For this review, take the finished solid that the model builds, in its own axes (mm). Coordinates: 2 decimals unless noted, no trailing zeros. Loops run counter-clockwise (first coordinate to the right, second up) from the corner with the lowest first, then second, coordinate; pieces in that order, holes last.
1. Take a section at C-C, the plane x = 12. State the section outline as (y, z) points.
2. Take a section at A-A, the plane x = -12.7. State the section outline as (y, z) points.
3. Clearance check with a flat-ended pin moving along its axis: P1, Ø5, axis at x = -12.7, y = -23.3, coming from the +Z side. State where the tip first meets the part, or that it passes through.
4. Take a section at B-B, the plane z = 1.9. State the section outline as (x, y) points, then the cut area to 3 significant figures.
5. To check wall thickness, follow probe 1 along Y at (x, z) = (-12.7, 1.7); probe 2 along X at (y, z) = (24, 2.3). State the ranges of each line that lie inside material, in increasing order.
Autodesk Inventor part; units mm, degrees
ref_plane "YZ Plane" through (0, 0, 0) normal (1, 0, 0) x (0, 1, 0)
ref_plane "XZ Plane" through (0, 0, 0) normal (0, 1, 0) x (-1, 0, 0)
ref_plane "XY Plane" through (0, 0, 0) normal (0, 0, 1) x (1, 0, 0)
sketch "Sketch1" plane through (0, 0, 0) normal (0, 0, 1) x (1, 0, 0)
  line L0 (-19.05, -36.0045) -> (19.05, -36.0045)
  line L1 (19.05, -36.0045) -> (19.05, 36.0045)
  line L2 (19.05, 36.0045) -> (-19.05, 36.0045)
  line L3 (-19.05, 36.0045) -> (-19.05, -36.0045)
  line L4 (-19.05, -36.0045) -> (19.05, 36.0045) construction
  line L5 (19.05, -36.0045) -> (-19.05, 36.0045) construction
  point P0 (0, 0)
  dimension "d0" = 38.1
  dimension "d1" = 72.009
extrude "Extrusion1" add sketch "Sketch1" along normal blind 2.54
sketch "Sketch2" plane through (0, 0, 2.54) normal (0, 0, 1) x (1, 0, 0)
  circle A0 centre (-12.7, 23.3045) radius 1.85
  circle A1 centre (12.7, 23.3045) radius 1.85
  circle A2 centre (-12.7, -23.3045) radius 1.85
  circle A3 centre (12.7, -23.3045) radius 1.85
  point P0 (0, 0)
extrude "Extrusion2" cut sketch "Sketch2" against normal blind 2.54
properties part number "GearPlate"
Results list:
1. outline: (-36, 0) - (-25.02, 0) - (-25.02, 2.54) - (-36, 2.54) - close; (-21.59, 0) - (21.59, 0) - (21.59, 2.54) - (-21.59, 2.54) - close; (25.02, 0) - (36, 0) - (36, 2.54) - (25.02, 2.54) - close
2. outline: (-36, 0) - (-25.15, 0) - (-25.15, 2.54) - (-36, 2.54) - close; (-21.45, 0) - (21.45, 0) - (21.45, 2.54) - (-21.45, 2.54) - close; (25.15, 0) - (36, 0) - (36, 2.54) - (25.15, 2.54) - close
3. P1: stops at z = 2.54
4. outline: (-19.05, -36) - (19.05, -36) - (19.05, 36) - (-19.05, 36) - close; hole circle Ø3.7 at (-12.7, -23.3); hole circle Ø3.7 at (-12.7, 23.3); hole circle Ø3.7 at (12.7, -23.3); hole circle Ø3.7 at (12.7, 23.3)
4. area: 2,700 mm2
5. probe 1: y = -36 to -25.15, -21.45 to 21.45, 25.15 to 36
5. probe 2: x = -19.05 to -14.41, -10.99 to 10.99, 14.41 to 19.05
